from build123d import *

# Parameters (mm, degrees)
SKETCH1_R           = 1.25
BOSS_EXTRUDE1_DEPTH = 3


with BuildPart() as part:
    # Sketch1 → Boss-Extrude1 (new body)
    with BuildSketch(Plane.XY.offset(11)):
        with BuildLine():
            Line((57.172491377, 74.714602367), (-57.172491341, 74.714602367))
            ThreePointArc((-57.172491341, 74.714602367), (-58.861466857, 74.05779571), (-59.662978082, 72.432491728))
            Line((-59.662978082, 72.432491728), (-65.762215507, 2.717889374))
            ThreePointArc((-65.762215507, 2.717889374), (-65.1149221, 0.811024486), (-63.271728747, 0))
            Line((-63.271728747, 0), (63.271728783, 0))
            ThreePointArc((63.271728783, 0), (65.114922137, 0.811024486), (65.762215543, 2.717889374))
            Line((65.762215543, 2.717889374), (59.662978119, 72.432491728))
            ThreePointArc((59.662978119, 72.432491728), (58.861466894, 74.05779571), (57.172491377, 74.714602367))
        make_face()
        with Locations((55.797994598, 70.714602357)):
            Circle(SKETCH1_R, mode=Mode.SUBTRACT)
        with Locations((-61.634765996, 4)):
            Circle(SKETCH1_R, mode=Mode.SUBTRACT)
        with Locations((-55.797994598, 70.714602357)):
            Circle(SKETCH1_R, mode=Mode.SUBTRACT)
        with Locations((61.634765996, 4)):
            Circle(SKETCH1_R, mode=Mode.SUBTRACT)
        with BuildLine():
            Line((53.217813713, 54.311351811), (56.268264715, 19.444537378))
            ThreePointArc((56.268264715, 19.444537378), (47.177875152, 8.611032956), (36.34437073, 17.701422518))
            Line((36.34437073, 17.701422518), (33.293919727, 52.56823695))
            ThreePointArc((33.293919727, 52.56823695), (42.38430929, 63.401741373), (53.217813713, 54.311351811))
        make_face(mode=Mode.SUBTRACT)
        with BuildLine():
            Line((-33.293919727, 52.56823695), (-36.34437073, 17.701422518))
            ThreePointArc((-36.34437073, 17.701422518), (-47.17787515, 8.611032957), (-56.268264712, 19.444537376))
            Line((-56.268264712, 19.444537376), (-53.217813716, 54.311351809))
            ThreePointArc((-53.217813716, 54.311351809), (-42.384309292, 63.401741375), (-33.293919727, 52.56823695))
        make_face(mode=Mode.SUBTRACT)
    extrude(amount=-BOSS_EXTRUDE1_DEPTH)


solid = part.part
CAD build for the part. Positions are in the model's coordinates, mm. A direction names the side the tool comes from. Give positions to 0.01 mm unless a question says otherwise; leave off trailing zeros. Write each loop counter-clockwise with the first axis right and the second up, starting at its lowest first coordinate (ties: lowest second). Pieces come first, ordered by that corner, then holes. Notation, with made-up numbers: (-19.5, 34) - (24.5, 34) arc R20 ccw to (24.5, 72) - close; hole circle Ø7 at (40.25, 85). An arc over 180 degrees is marked (long way). Answer as CSV lines item,"result".
Q1. Flat gauge pins, fed straight in: pin 1 Ø1 at (y, z) = (64, 8.5) entering from +X; pin 2 Ø2 at (x, y) = (-55.8, 70.71) entering from +Z. Where does each tip first touch, or does it go through?
Result set:
pin 1,"x = 60.44"
pin 2,"through"
Q2. 3-axis set-ups, long thin cutter, end or side, ignore diameter. For faces 4 (the face through (-54.764, 36.634, 9.521)), 5 (the face through (-1, 38, 11)): which of +Z, -Z, +X, -X, +Y, -Y reach the whole face in a straight line?
Result set:
face 4,"+Z, -Z"
face 5,"+Z, +X, -X, +Y, -Y"
Q3. Band-saw the part on C-C (z = 10.35). Give the cut face in (x, y), and give its area (3 significant figures).
Result set:
outline,"(-65.76, 2.72) arc R2.5 ccw to (-63.27, 0) - (63.27, 0) arc R2.5 ccw to (65.76, 2.72) - (59.66, 72.43) arc R2.5 ccw to (57.17, 74.71) - (-57.17, 74.71) arc R2.5 ccw to (-59.66, 72.43) - close; hole circle Ø2.5 at (-61.63, 4); hole circle Ø2.5 at (-55.8, 70.71); hole (-56.27, 19.44) arc R10 ccw to (-36.34, 17.7) - (-33.29, 52.57) arc R10 ccw to (-53.22, 54.31) - close; hole (33.29, 52.57) - (36.34, 17.7) arc R10 ccw to (56.27, 19.44) - (53.22, 54.31) arc R10 ccw to start; hole circle Ø2.5 at (55.8, 70.71); hole circle Ø2.5 at (61.63, 4)"
area,"7,320 mm²"
Q4. Band-saw the part on A-A (y = 50.5). Give the cut face in (x, z).
Result set:
outline,"(-61.58, 8) - (-53.55, 8) - (-53.55, 11) - (-61.58, 11) - close; (-33.47, 8) - (33.47, 8) - (33.47, 11) - (-33.47, 11) - close; (53.55, 8) - (61.58, 8) - (61.58, 11) - (53.55, 11) - close"
Q5. Drill centre lines: line 1 (X direction, y = 56.5, z = 10.45); line 2 (X direction, y = 10.5, z = 10.25); line 3 (Y direction, x = 48, z = 8.6). Where is each one in solid material? Low to high. Write a range as from..to.
Result set:
line 1,"-61.06..-52.78, -33.74..33.74, 52.78..61.06"
line 2,"-65.08..-52.21, -40.4..40.4, 52.21..65.08"
line 3,"0..8.72, 62.24..74.71"
Q6. Band-saw the part on B-B (x = 49.5). Give the cut face in (y, z).
Result set:
outline,"(0, 8) - (9.1, 8) - (9.1, 11) - (0, 11) - close; (61.25, 8) - (74.71, 8) - (74.71, 11) - (61.25, 11) - close"
Q7. Pull direction Y, two halves, no side cores. Call faces 1 (the face through (62.755, 37.087, 9.521)), 2 (the face through (-1, 38, 8)), 3 (the face through (34.84, 34.89, 9.52)): released by +Y, released by -Y, zero draft, split by the parting line, or undercut.
Result set:
face 1,"released by +Y"
face 2,"zero draft"
face 3,"undercut"
Q8. Band-saw the part on D-D (y = 29). Give the cut face in (x, z), and give its area (3 significant figures).
Result set:
outline,"(-63.46, 8) - (-55.43, 8) - (-55.43, 11) - (-63.46, 11) - close; (-35.36, 8) - (35.36, 8) - (35.36, 11) - (-35.36, 11) - close; (55.43, 8) - (63.46, 8) - (63.46, 11) - (55.43, 11) - close"
area,"260 mm²"
